CAD build for the part. Positions are in the model's coordinates, mm. Face numbers are marked on the shaded views. A direction names the side the tool comes from. Give positions to 0.01 mm unless a question says otherwise; leave off trailing zeros. Write each loop counter-clockwise with the first axis right and the second up, starting at its lowest first coordinate (ties: lowest second). Pieces come first, ordered by that corner, then holes. Notation, with made-up numbers: (85.25, 11.5) - (117.25, 11.5) arc R16 ccw to (117.25, 34.5) - close; hole circle Ø4 at (77.5, 84). An arc over 180 degrees is marked (long way). Answer as a JSON object with one key per item and string values.
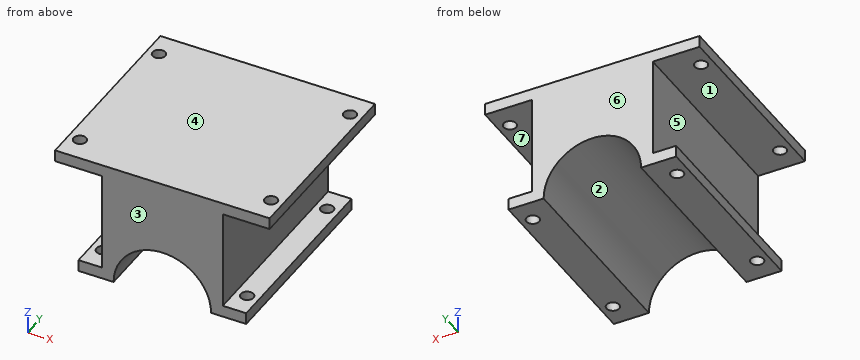
from build123d import *

# Parameters (mm, degrees)
BOSS_EXTRU_2_DEPTH      = 50
ESQUISSE2_R             = 1.625
ENL_V_MAT_EXTRU_2_DEPTH = 6
ESQUISSE4_R             = 1.625
ENL_V_MAT_EXTRU_3_DEPTH = 14
ESQUISSE3_R             = 1.625
ENL_V_MAT_EXTRU_4_DEPTH = 14


with BuildPart() as part:
    # Esquisse1 → Boss.-Extru.2 (new body)
    with BuildSketch(Plane(origin=(0, 0, 0), x_dir=(1, 0, 0), z_dir=(0, 1, 0))):
        with BuildLine():
            Line((-6, 28.5), (-6, 31.5))
            Line((-6, 31.5), (3, 31.5))
            ThreePointArc((3, 31.5), (15.5, 19), (28, 31.5))
            Line((28, 31.5), (37, 31.5))
            Line((37, 31.5), (37, 28.5))
            Line((37, 28.5), (31, 28.5))
            Line((31, 28.5), (31, 3))
            Line((31, 3), (43, 3))
            Line((43, 3), (43, 0))
            Line((43, 0), (-12, 0))
            Line((-12, 0), (-12, 3))
            Line((-12, 3), (0, 3))
            Line((0, 3), (0, 28.5))
            Line((0, 28.5), (-6, 28.5))
        make_face()
    extrude(amount=BOSS_EXTRU_2_DEPTH)

    # Esquisse2 → Enlèv. mat.-Extru.2 (cut)
    with BuildSketch(Plane(origin=(0, 0, -31.5), x_dir=(-1, 0, 0), z_dir=(0, 0, -1))):
        with Locations((3, 44)):
            Circle(ESQUISSE2_R)
        with Locations((3, 6)):
            Circle(ESQUISSE2_R)
        with Locations((-34, 44)):
            Circle(ESQUISSE2_R)
        with Locations((-34, 6)):
            Circle(ESQUISSE2_R)
    extrude(amount=-ENL_V_MAT_EXTRU_2_DEPTH, mode=Mode.SUBTRACT)

    # Esquisse4 → Enlèv. mat.-Extru.3 (cut)
    with BuildSketch(Plane(origin=(0, 0, -3), x_dir=(-1, 0, 0), z_dir=(0, 0, -1))):
        with Locations((9, 6.25)):
            Circle(ESQUISSE4_R)
        with Locations((9, 43.75)):
            Circle(ESQUISSE4_R)
    extrude(amount=-ENL_V_MAT_EXTRU_3_DEPTH, mode=Mode.SUBTRACT)

    # Esquisse3 → Enlèv. mat.-Extru.4 (cut)
    with BuildSketch(Plane(origin=(0, 0, -3), x_dir=(-1, 0, 0), z_dir=(0, 0, -1))):
        with Locations((-40, 6.25)):
            Circle(ESQUISSE3_R)
        with Locations((-40, 43.75)):
            Circle(ESQUISSE3_R)
    extrude(amount=-ENL_V_MAT_EXTRU_4_DEPTH, mode=Mode.SUBTRACT)


solid = part.part
Item 1: Flat gauge pins, fed straight in: P1, Ø4, axis at x = 13.5, y = 15, coming from the -Z side; P2, Ø6, axis at y = 5, z = -14, coming from the -X side; P3, Ø4, axis at x = 40, y = 6.25, coming from the -Z side. Where does each tip first touch, or does it go through?
Entries:
{"P1": "z = -19.66", "P2": "x = 0", "P3": "z = -3"}
Item 2: Cut at B-B (x = -3). Give the cut face in (y, z) (3 decimals), and give its area (4 significant figures).
Entries:
{"outline": "(0, -31.5) - (4.375, -31.5) - (4.375, -28.5) - (0, -28.5) - close; (0, -3) - (50, -3) - (50, 0) - (0, 0) - close; (7.625, -31.5) - (42.375, -31.5) - (42.375, -28.5) - (7.625, -28.5) - close; (45.625, -31.5) - (50, -31.5) - (50, -28.5) - (45.625, -28.5) - close", "area": "280.5 mm2"}
Item 3: Cut at C-C (z = -24.5). Give the cut face in (x, y), and give its area (3 significant figures).
Entries:
{"outline": "(0, 0) - (5.14, 0) - (5.14, 50) - (0, 50) - close; (25.86, 0) - (31, 0) - (31, 50) - (25.86, 50) - close", "area": "514 mm2"}
Item 4: Probe line 1 (Y direction, x = 34, z = -29.95) (3 decimals); line 2 (Y direction, x = 40, z = -1.85) (3 decimals); line 3 (Z direction, x = 35, y = 28). List the from-to ranges inside material, lowest first. Write a range as from..to.
Entries:
{"line 1": "0..4.375, 7.625..42.375, 45.625..50", "line 2": "0..4.625, 7.875..42.125, 45.375..50", "line 3": "-31.5..-28.5, -3..0"}
Item 5: Cut at D-D (y = 9.5). Give the cut face in (x, z), and give its area (3 significant figures).
Entries:
{"outline": "(-12, -3) - (0, -3) - (0, -28.5) - (-6, -28.5) - (-6, -31.5) - (3, -31.5) arc R12.5 cw to (28, -31.5) - (37, -31.5) - (37, -28.5) - (31, -28.5) - (31, -3) - (43, -3) - (43, 0) - (-12, 0) - close", "area": "839 mm2"}
Item 6: Mould opens along Z. For the marked faces 1, 2, 3 and 4 say: +Z half, -Z half, draft (parallel to the pull), parting line (faces both ways), or undercut.
Entries:
{"face 1": "undercut", "face 2": "-Z half", "face 3": "draft", "face 4": "+Z half"}
Item 7: Cut at A-A (x = 40). Give the cut face in (y, z) (3 decimals), and give its area (4 significant figures).
Entries:
{"outline": "(0, -3) - (4.625, -3) - (4.625, 0) - (0, 0) - close; (7.875, -3) - (42.125, -3) - (42.125, 0) - (7.875, 0) - close; (45.375, -3) - (50, -3) - (50, 0) - (45.375, 0) - close", "area": "130.5 mm2"}
Item 8: Which spindle directions (+Z, -Z, +X, -X, +Y, -Y) get a long thin tool onto all of the face, cutting with end or side? Do the marked faces 5, 6 and 7. Say none if no direction does.
Entries:
{"face 5": "-X, +Y, -Y", "face 6": "+Z, -Z, +X, -X, +Y", "face 7": "+X, +Y, -Y"}
